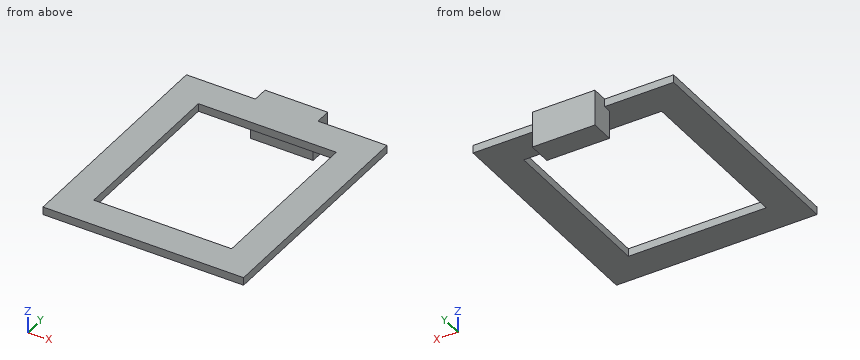
from build123d import *

# Parameters (mm, degrees)
F3_W     = 128
F3_H     = 148
F3_W_2   = 88
F3_H_2   = 108
F4_DEPTH = 5
F5_W     = 40
F5_H     = 5
F6_DEPTH = 10
F7_W     = 40
F7_H     = 10
F8_DEPTH = 18
F9_DEPTH = 5


with BuildPart() as f4:
    # F3 (on Top) → F4 (new body)
    with BuildSketch(Plane.XY):
        Rectangle(F3_W, F3_H)
        Rectangle(F3_W_2, F3_H_2, mode=Mode.SUBTRACT)
    extrude(amount=F4_DEPTH)

    # F5 (on face) → F6 (join)
    with BuildSketch(Plane(origin=(0, 74, 0), x_dir=(-1, 0, 0), z_dir=(0, 1, 0))):
        with Locations((0, 2.5)):
            Rectangle(F5_W, F5_H)
    extrude(amount=F6_DEPTH)

    # F7 (on face) → F8 (join)
    with BuildSketch(Plane(origin=(0, 0, 0), x_dir=(1, 0, 0), z_dir=(0, 0, -1))):
        with Locations((0, -79)):
            Rectangle(F7_W, F7_H)
    extrude(amount=F8_DEPTH)

    # F9 (add): a face of the model
    f9_faces = [f4.faces().sort_by_distance(p)[0] for p in [
        (0, 74, -9),
    ]]
    extrude(f9_faces, amount=F9_DEPTH)


solid = f4.part
Model file for the job. Use its own axes, mm. Coordinates: 2 decimals unless noted, no trailing zeros. Write each loop counter-clockwise with the first axis right and the second up, starting at its lowest first coordinate (ties: lowest second). Pieces come first, ordered by that corner, then holes. Notation, with made-up numbers: (38, 65.5) -> (57, 65.5) arc R25 cw to (57, 81.5) -> close; hole circle Ø1 at (84, -24). An arc over 180 degrees is marked (long way). One line per item, written item: value. Start each with the question number.
1) Slice it at B-B on y = -2. Write the cut outline in (x, z), then the cut area to 3 significant figures.
2) Probe probe 1 along X at (y, z) = (6.5, 1.5); probe 2 along Y at (x, z) = (4, 1); probe 3 along Z at (x, y) = (-26.5, 71.5). List the from-to ranges inside material, lowest first.
3) Flat gauge pins, fed straight in: pin 1 Ø5 at (x, y) = (47.5, -36) entering from -Z; pin 2 Ø4 at (x, z) = (-37, 3.5) entering from +Y; pin 3 Ø9 at (x, z) = (5.5, -13) entering from -Y; pin 4 Ø8 at (x, y) = (37, -41) entering from -Z. Where does each tip first touch, or does it go through?
4) Slice it at A-A on x = -41. Write the cut outline in (y, z).
5) Slice it at C-C on x = 17. Write the cut outline in (y, z), then the cut area to 3 significant figures.
6) Slice it at D-D on z = -10. Write the cut outline in (x, y).
Answers follow:
1. outline: (-64, 0) -> (-44, 0) -> (-44, 5) -> (-64, 5) -> close; (44, 0) -> (64, 0) -> (64, 5) -> (44, 5) -> close
1. area: 200 mm2
2. probe 1: -64 to -44, 44 to 64
2. probe 2: -74 to -54, 54 to 84
2. probe 3: 0 to 5
3. pin 1: z = 0
3. pin 2: y = 74
3. pin 3: y = 69
3. pin 4: through
4. outline: (-74, 0) -> (-54, 0) -> (-54, 5) -> (-74, 5) -> close; (54, 0) -> (74, 0) -> (74, 5) -> (54, 5) -> close
5. outline: (-74, 0) -> (-54, 0) -> (-54, 5) -> (-74, 5) -> close; (54, 0) -> (69, 0) -> (69, -18) -> (84, -18) -> (84, 5) -> (54, 5) -> close
5. area: 520 mm2
6. outline: (-20, 69) -> (20, 69) -> (20, 84) -> (-20, 84) -> close
